```python
from build123d import *

# Parameters (mm, degrees)
SKETCH1_W           = 100
SKETCH1_H           = 75
BOSS_EXTRUDE1_DEPTH = 1
SKETCH2_W           = 1
SKETCH2_H           = 73
BOSS_EXTRUDE2_DEPTH = 60


with BuildPart() as part:
    # Sketch1 → Boss-Extrude1 (new body)
    with BuildSketch(Plane.XY):
        with Locations((50, 37.5)):
            Rectangle(SKETCH1_W, SKETCH1_H)
    extrude(amount=BOSS_EXTRUDE1_DEPTH)

    # Sketch2 → Boss-Extrude2 (add)
    with BuildSketch(Plane.XY.offset(1)):
        Polygon((100, 75), (0, 75), (0, 74), (1, 74), (99, 74), (100, 74), align=None)
        with Locations((0.5, 37.5)):
            Rectangle(SKETCH2_W, SKETCH2_H)
        Polygon((1, 1), (0, 1), (0, 0), (99, 0), (99, 1), align=None)
        Polygon((100, 0), (100, 74), (99, 74), (99, 1), (99, 0), align=None)
    extrude(amount=BOSS_EXTRUDE2_DEPTH)


solid = part.part
```
CAD build for the part. Positions are in the model's coordinates, mm. A direction names the side the tool comes from. Give positions to 0.01 mm unless a question says otherwise; leave off trailing zeros. Write each loop counter-clockwise with the first axis right and the second up, starting at its lowest first coordinate (ties: lowest second). Pieces come first, ordered by that corner, then holes. Notation, with made-up numbers: (60, -37.5) -> (105, -37.5) arc R27 cw to (105, -4.5) -> close; hole circle Ø7 at (11.5, 38). An arc over 180 degrees is marked (long way). Write each question's results on one line, items separated by ' | '.
1. Two-plate mould, pull along Y, no slides. Class faces 3 (the flat face through (99, 38, 31)), 4 (the flat face through (49, 0, 30)), 5 (the flat face through (49, 38, 0)): pulls with the +Y half, pulls with the -Y half, needs draft (parallel to the pull), parting line crosses it, or undercut.
Geometry check:
face 3: undercut | face 4: pulls with the -Y half | face 5: needs draft
2. Which spindle directions (+Z, -Z, +X, -X, +Y, -Y) get a long thin tool onto all of the face, cutting with end or side? Do faces 1 (the flat face through (51, 75, 30)), 2 (the flat face through (49, 74, 31)). Say none if no direction does.
Geometry check:
face 1: +Z, -Z, +X, -X, +Y | face 2: +Z
3. Wall check: probe 1 along X at (y, z) = (52.5, 36.5); probe 2 along Y at (x, z) = (38.5, 38); probe 3 along Z at (x, y) = (86, 67). Give the ranges that are in metal, low to high. Write a range as [from, to].
Geometry check:
probe 1: [0, 1], [99, 100] | probe 2: [0, 1], [74, 75] | probe 3: [0, 1]
4. Drop a flat-ended pin along its axis: P1, Ø10, axis at x = 60.5, y = 24, coming from the +Z side. Give the stop position or say it passes through.
Geometry check:
P1: z = 1
5. Cut at A-A, the plane z = 36. Write the cut outline in (x, y).
Geometry check:
outline: (0, 0) -> (100, 0) -> (100, 75) -> (0, 75) -> close; hole (1, 1) -> (99, 1) -> (99, 74) -> (1, 74) -> close
6. Cut at B-B, the plane y = 52. Write the cut outline in (x, z), then the cut area to 3 significant figures.
Geometry check:
outline: (0, 0) -> (100, 0) -> (100, 61) -> (99, 61) -> (99, 1) -> (1, 1) -> (1, 61) -> (0, 61) -> close | area: 220 mm²
7. Cut at C-C, the plane x = 58. Write the cut outline in (y, z), then the cut area to 3 significant figures.
Geometry check:
outline: (0, 0) -> (75, 0) -> (75, 61) -> (74, 61) -> (74, 1) -> (1, 1) -> (1, 61) -> (0, 61) -> close | area: 195 mm²
